Part print with two shaded views. Sizes in mm from the minimum x, y, z corner. Coordinates: 2 decimals unless noted, no trailing zeros. Loops run counter-clockwise (first coordinate to the right, second up) from the corner with the lowest first, then second, coordinate; pieces in that order, holes last. Notation, with made-up numbers: M -7.75,29.5 L 42.25,29.5 A31 ccw 42.25,55.5 Z; hole C 12,27 d11. An arc over 180 degrees is marked long. Write item = value, one per line. Start each with the question number.
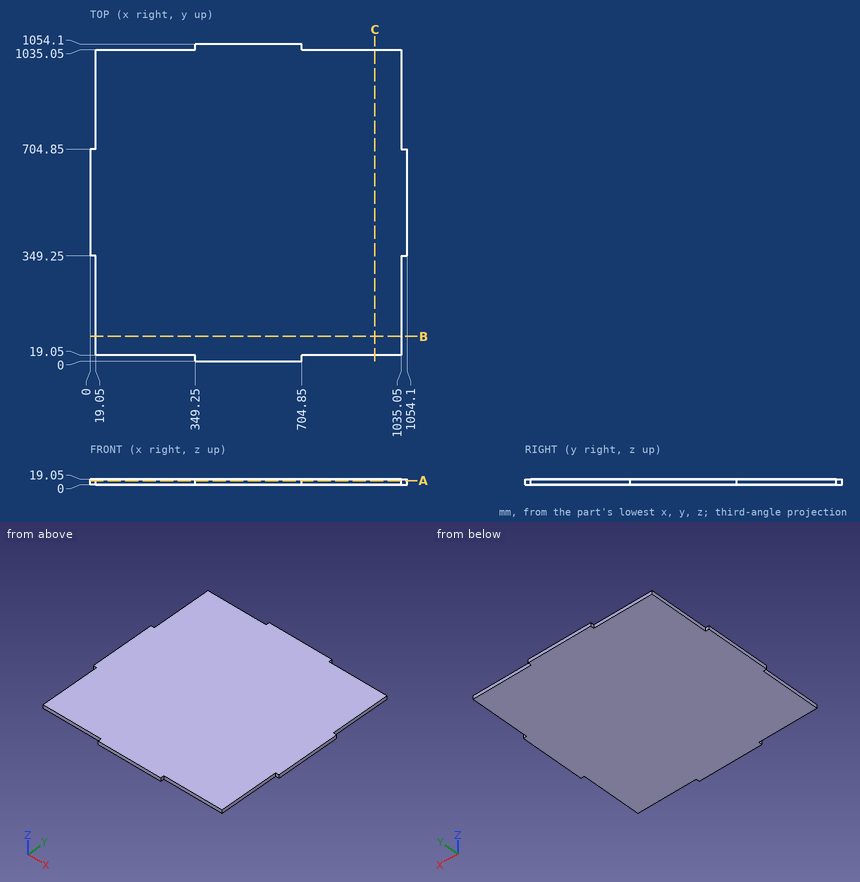
Item 1: Pin check, flat tips, straight feed: pin 1 Ø5 at (y, z) = (809, 14) entering from +X; pin 2 Ø9.5 at (x, z) = (941, 9.5) entering from +Y; pin 3 Ø9.5 at (x, z) = (1040.5, 5.5) entering from -Y. Stop position of each tip, or through.
Item 2: Probe L1, parallel to Y at x = 764, z = 13.5. List the from-to ranges inside material, lowest first.
Item 3: Cut at A-A (z = 13.5). Give the cut face in (x, y).
Item 4: Cut at B-B (y = 81.5). Give the cut face in (x, z).
Reported:
q1.pin_1 = 1035.05
q1.pin_2 = 1035.05
q1.pin_3 = 349.25
q2.L1 = 19.05 to 1035.05
q3.outline = M 0,349.25 L 19.05,349.25 L 19.05,19.05 L 349.25,19.05 L 349.25,0 L 704.85,0 L 704.85,19.05 L 1035.05,19.05 L 1035.05,349.25 L 1054.1,349.25 L 1054.1,704.85 L 1035.05,704.85 L 1035.05,1035.05 L 704.85,1035.05 L 704.85,1054.1 L 349.25,1054.1 L 349.25,1035.05 L 19.05,1035.05 L 19.05,704.85 L 0,704.85 Z
q4.outline = M 19.05,0 L 1035.05,0 L 1035.05,19.05 L 19.05,19.05 Z
